Verification items for the finished model (mm, model axes). Give positions to 0.01 mm unless a question says otherwise; leave off trailing zeros. Order: outer loops, then holes, each group sorted by start corner. A loop starts at its lowest first (then second) coordinate and runs counter-clockwise, first axis right, second up. Notation, with made-up numbers: (18, 25.25) -> (38, 25.25) arc R21 ccw to (38, 46.25) -> close; hole circle Ø7 at (-11, 66). An arc over 180 degrees is marked (long way). Return JSON: item names as keys, results as strings. Group by question number.
(1) Cross-section at A-A on z = 393. Enter the section's corners in (x, y), then the cut area to 3 significant figures.
(2) Depth check by flat-ended pin: pin 1 Ø5 at (x, y) = (0, 0) entering from +Z; pin 2 Ø5 at (x, y) = (-7.5, -1.5) entering from -Z. Enter the tip coordinate at first touch or a pass-through.
(3) Thickness scan on line 1 along Y through (x, z) = (0, 135); line 2 along Y through (x, z) = (2.5, 368). Record the ranges inside material, lowest first.
from build123d import *

# Parameters (mm, degrees)
F0_W     = 40
F0_H     = 40
F1_DEPTH = 573.5
F3_D     = 8
F4_R     = 4


with BuildPart() as f1:
    # F0 (on Top) → F1 (new body)
    with BuildSketch(Plane.XY):
        Rectangle(F0_W, F0_H)
    extrude(amount=F1_DEPTH)

    # F3 (through all)
    with Locations(Plane.XY.offset(573.5)):
        with Locations((0, 0)):
            Hole(F3_D / 2)

    # F4
    f4_edges = [f1.edges().sort_by_distance(p)[0] for p in [
        (-20, -20, 286.75),
        (20, -20, 286.75),
        (20, 20, 286.75),
        (-20, 20, 286.75),
    ]]
    fillet(f4_edges, radius=F4_R)


solid = f1.part
Verdict:
{
 "1": {"outline": "(-20, -16) arc R4 ccw to (-16, -20) -> (16, -20) arc R4 ccw to (20, -16) -> (20, 16) arc R4 ccw to (16, 20) -> (-16, 20) arc R4 ccw to (-20, 16) -> close; hole circle Ø8 at (0, 0)", "area": "1,540 mm²"},
 "2": {"pin 1": "through", "pin 2": "z = 0"},
 "3": {"line 1": "-20 to -4, 4 to 20", "line 2": "-20 to -3.12, 3.12 to 20"}
}
